```python
from build123d import *

# Parameters (mm, degrees)
F0_W        = 170.942
F0_H        = 120.142
F1_DEPTH    = 12.7
F2_W        = 184.658
F2_H        = 133.858
F2_W_2      = 170.942
F2_H_2      = 120.142
F3_DEPTH    = 6.35
F4_T        = 3.81
F4_T3_DEPTH = 127.762
F4_T5_DEPTH = 178.562


# Not quite as in the source:
# - a shell that OpenCascade refuses in one call is made with other operations: the cavity is built on its own and cut out


with BuildPart() as f1:
    # F0 (on Front) → F1 (new body)
    with BuildSketch(Plane.XZ):
        with Locations((85.471, 60.071)):
            Rectangle(F0_W, F0_H)
    extrude(amount=F1_DEPTH)

    # F2 (on face) → F3 (join)
    with BuildSketch(Plane.XZ.offset(12.7)):
        with Locations((85.471, 60.071)):
            Rectangle(F2_W, F2_H)
        with Locations((85.471, 60.071)):
            Rectangle(F2_W_2, F2_H_2, mode=Mode.SUBTRACT)
    extrude(amount=-F3_DEPTH)

    # F4: shell of thickness 3.81, made by hand


with BuildPart() as f4_core1:
    # F4_t2: copy of F1
    add(f1.part)

    # the walls: a layer under each face that stays
    f4_faces = [f4_core1.faces().sort_by_distance(p)[0] for p in [
        (0, -3.175, 60.071),
        (85.471, -3.175, 0),
        (-0.7027333333, -6.35, -2.3960666667),
        (85.471, -3.175, 120.142),
        (170.942, -3.175, 60.071),
        (-6.858, -9.525, 60.071),
        (85.471, -9.525, -6.858),
        (177.8, -9.525, 60.071),
        (85.471, -9.525, 127),
        (85.471, -12.7, 60.071),
    ]]
    thicken(f4_faces, amount=-F4_T, mode=Mode.SUBTRACT)

    # F4_s4 → F4_t3 (cut)
    with BuildSketch(Plane.XY.offset(-3.81)):
        Polygon((-0.0381, -6.3119), (3.81, -6.35), (3.81, -10.16), (0, -10.16), align=None)
        Polygon((170.9801, -6.3119), (170.942, -10.16), (167.132, -10.16), (167.132, -6.35), align=None)
    extrude(amount=F4_T3_DEPTH, mode=Mode.SUBTRACT)

    # F4_s6 → F4_t5 (cut)
    with BuildSketch(Plane.YZ.offset(-3.81)):
        Polygon((-6.3119, -0.0381), (-6.35, 3.81), (-10.16, 3.81), (-10.16, 0), align=None)
        Polygon((-6.3119, 120.1801), (-10.16, 120.142), (-10.16, 116.332), (-6.35, 116.332), align=None)
    extrude(amount=F4_T5_DEPTH, mode=Mode.SUBTRACT)


with BuildPart() as f1_1:
    add(f1.part)

    # what is left inside the walls is the cavity
    f4_cavity = [f4_core1.part.solids().sort_by_distance(p)[0] for p in [
        (85.471, -8.8519, 41.317333),
    ]]
    add(f4_cavity, mode=Mode.SUBTRACT)


solid = f1_1.part
```
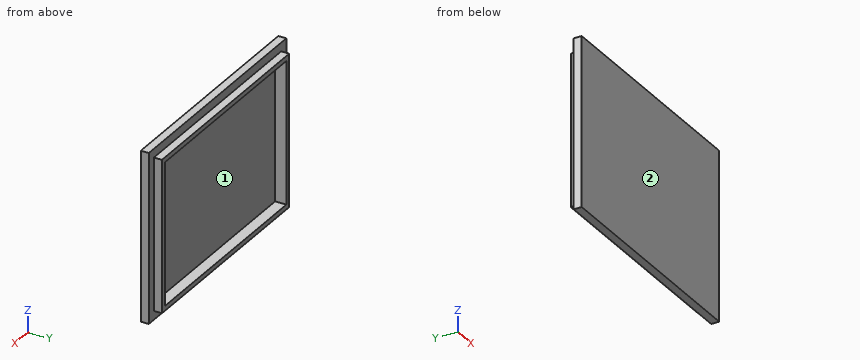
Could you check a few things on this model? Use its own coordinates, in mm. Face numbers are marked on the shaded views. Round coordinates to 2 decimals unless told otherwise and drop trailing zeros. Loops run counter-clockwise (first coordinate to the right, second up) from the corner with the lowest first, then second, coordinate; pieces in that order, holes last. Notation, with made-up numbers: (48.5, -11) - (65.5, -11) arc R7 ccw to (65.5, -7) - close; hole circle Ø11 at (81.5, 70). An arc over 180 degrees is marked (long way). Answer as CSV lines item,"result".
1. I want a section at C-C on x = 131. List the corners of the cut face in (y, z) for me.
Filled in:
outline,"(-12.7, -6.86) - (-6.35, -6.86) - (-6.35, 0) - (0, 0) - (0, 3.81) - (-8.89, 3.81) - (-8.89, 116.33) - (0, 116.33) - (0, 120.14) - (-6.35, 120.14) - (-6.35, 127) - (-12.7, 127) - close"
2. We'd pull the mould along Z, two halves only. Please class the marked faces 1 and 2: +Z half, -Z half, draft (parallel to the pull), parting line (faces both ways), or undercut.
Filled in:
face 1,"undercut"
face 2,"draft"
3. For pin 1 Ø8 at (x, z) = (90, 55) entering from +Y; pin 2 Ø3 at (x, y) = (71, -2) entering from -Z; pin 3 Ø4.5 at (y, z) = (-2.5, 44.5) entering from -X, each with a flat end and sliding along its axis, tell me the tip position at first contact or that it passes through.
Filled in:
pin 1,"stops at y = -8.89"
pin 2,"stops at z = 0"
pin 3,"stops at x = 0"
4. I want a section at B-B on z = 100. List the corners of the cut face in (x, y) for me.
Filled in:
outline,"(-6.86, -12.7) - (177.8, -12.7) - (177.8, -6.35) - (170.94, -6.35) - (170.94, 0) - (167.13, 0) - (167.13, -8.89) - (3.81, -8.89) - (3.81, 0) - (0, 0) - (0, -6.35) - (-6.86, -6.35) - close"
5. Please list where these lines run through material, in increasing order: line 1 along Z through (x, y) = (13, -4.5); line 2 along X through (y, z) = (-4.75, 80); line 3 along Z through (x, y) = (72, -8.5). Write a range as [from, to].
Filled in:
line 1,"z = [0, 3.81], [116.33, 120.14]"
line 2,"x = [0, 3.81], [167.13, 170.94]"
line 3,"z = [-6.86, 3.81], [116.33, 127]"
6. I want a section at A-A on y = -3.5. List the corners of the cut face in (x, z) for me, then the cut area to 3 significant figures.
Filled in:
outline,"(0, 0) - (170.94, 0) - (170.94, 120.14) - (0, 120.14) - close; hole (3.81, 3.81) - (167.13, 3.81) - (167.13, 116.33) - (3.81, 116.33) - close"
area,"2,160 mm^2"
